from build123d import *

# Parameters (mm, degrees)
F1_DEPTH = 25.4
F2_W     = 46.1691659327
F2_H     = 29.3826218694
F3_DEPTH = 19.05
F5_DEPTH = 25.4


with BuildPart() as f1:
    # F0 (on Top) → F1 (new body)
    with BuildSketch(Plane.XY):
        Polygon((70.5610662699, 62.708877027), (19.1396083683, 62.708877027), (19.1396083683, 30.9927258641), (22.5176624954, 30.9927258641), (68.1213587523, 30.9927258641), (70.5610662699, 30.9927258641), align=None)
    extrude(amount=F1_DEPTH)

    # F2 (on face) → F3 (cut)
    with BuildSketch(Plane(origin=(0, 0, 0), x_dir=(1, 0, 0), z_dir=(0, 0, -1))):
        with Locations((44.8503373191, -45.6840367988)):
            Rectangle(F2_W, F2_H)
    extrude(amount=-F3_DEPTH, mode=Mode.SUBTRACT)

    # F4 (on face) → F5 (join)
    with BuildSketch(Plane(origin=(0, 0, 0), x_dir=(1, 0, 0), z_dir=(0, 0, -1))):
        Polygon((67.9349202854, -30.9927258641), (70.5610662699, -30.9927258641), (70.5610662699, -27.0810292719), (69.0370662699, -27.0810292719), align=None)
        Polygon((19.1396083683, -27.0810292719), (19.1396083683, -30.9927258641), (21.7657543527, -30.9927258641), (20.6636083683, -27.0810292719), align=None)
    extrude(amount=-F5_DEPTH)


solid = f1.part
Can you work these out from the model? Positions are in its coordinate system, mm. A direction names the side the tool comes from. Coordinates: 2 decimals unless noted, no trailing zeros. Order: outer loops, then holes, each group sorted by start corner. A loop starts at its lowest first (then second) coordinate and runs counter-clockwise, first axis right, second up. Notation, with made-up numbers: (45, -37) - (67, -37) arc R21 ccw to (67, -20) - close; hole circle Ø8 at (3.5, 69.25). An arc over 180 degrees is marked (long way). Answer as a JSON object with one key per item and string values. Group by question number.
Q1. Imagine slicing it at C-C (x = 42). Please give me the cut outline in (y, z), and give its area (3 significant figures).
Q2. I need wall thicknesses on line 1 (X direction, y = 43, z = 17.5); line 2 (Z direction, x = 34, y = 56); line 3 (Y direction, x = 24.5, z = 21.75). Which ranges of each line are inside material? Lowest first, please. Write a range as from..to.
Q3. On a 3-axis mill with a long thin cutter (end or side, diameter ignored), from which of +Z, -Z, +X, -X, +Y, -Y can I reach the whole of each face in a straight line? I mean faces 5 (the face through (21.22, 29.06, 12.52)), 6 (the face through (21.766, 46, 9)), 7 (the face through (45, 61, 0)). Say none if no direction works.
Q4. We'd pull the mould along X, two halves only. Please class faces 1 (the face through (70.561, 45, 13)), 2 (the face through (19.14, 45, 13)), 3 (the face through (45, 60.375, 9)), 4 (the face through (68.494, 29.009, 12.522)): +X half, -X half, draft (parallel to the pull), parting line (faces both ways), or undercut.
Q5. Imagine slicing it at A-A (y = 43.5). Please give me the cut outline in (x, z).
Q6. Imagine slicing it at B-B (z = 7.75). Please give me the cut outline in (x, y), and give its area (3 significant figures).
Q7. Will these pins go through, and if not, where does the flat tip stop? P1, Ø1.5, axis at x = 38.5, z = 13, coming from the -Y side; P2, Ø2, axis at x = 32, y = 40, coming from the -Z side; P3, Ø9.5, axis at x = 41, z = 14.5, coming from the -Y side.
Determined:
{
 "1": {"outline": "(30.99, 19.05) - (60.38, 19.05) - (60.38, 0) - (62.71, 0) - (62.71, 25.4) - (30.99, 25.4) - close", "area": "246 mm2"},
 "2": {"line 1": "x = 19.14..21.77, 67.93..70.56", "line 2": "z = 19.05..25.4", "line 3": "y = 30.99..62.71"},
 "3": {"face 5": "+Z, -Z, -Y", "face 6": "-Z, -Y", "face 7": "-Z, +X, -X, +Y, -Y"},
 "4": {"face 1": "+X half", "face 2": "-X half", "face 3": "undercut", "face 4": "undercut"},
 "5": {"outline": "(19.14, 0) - (21.77, 0) - (21.77, 19.05) - (67.93, 19.05) - (67.93, 0) - (70.56, 0) - (70.56, 25.4) - (19.14, 25.4) - close"},
 "6": {"outline": "(19.14, 27.08) - (20.66, 27.08) - (21.77, 30.99) - (21.77, 60.38) - (67.93, 60.38) - (67.93, 30.99) - (69.04, 27.08) - (70.56, 27.08) - (70.56, 62.71) - (19.14, 62.71) - close", "area": "291 mm2"},
 "7": {"P1": "stops at y = 60.38", "P2": "stops at z = 19.05", "P3": "stops at y = 30.99"}
}
